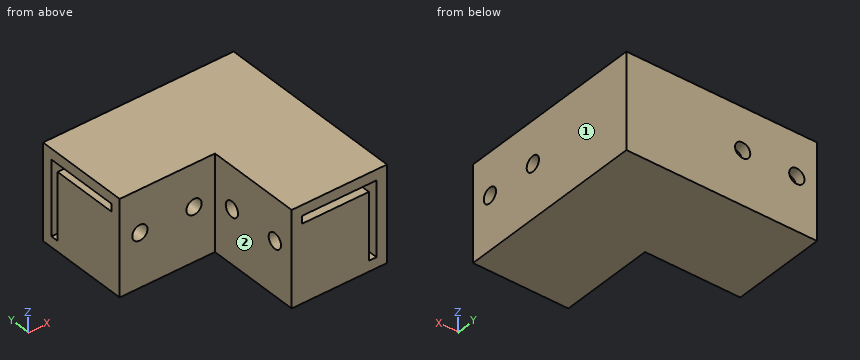
```python
from build123d import *

# Parameters (mm, degrees)
F0_W      = 25
F0_H      = 25
F1_DEPTH  = 25
F2_DEPTH  = 25
F3_DEPTH  = 25
F4_W      = 25
F4_H      = 25
F5_DEPTH  = 25
F6_W      = 17.5
F6_H      = 2
F6_W_2    = 2
F6_H_2    = 17.5
F7_DEPTH  = 25
F8_W      = 2
F8_H      = 2
F8_W_2    = 17.5
F8_H_2    = 17.5
F9_DEPTH  = 25
F10_R     = 2
F11_DEPTH = 25
F12_R     = 2
F13_DEPTH = 25


# Not quite as in the source:
# - a feature names something its author has since deleted; it is built from what else it names


with BuildPart() as f1:
    # F0 (on Top) → F1 (new body)
    with BuildSketch(Plane.XY):
        with Locations((12.5, 12.5)):
            Rectangle(F0_W, F0_H)
    extrude(amount=F1_DEPTH)

    # F2 (add): a face of the model
    f2_faces = [f1.faces().sort_by_distance(p)[0] for p in [
        (12.5, 0, 12.5),
    ]]
    extrude(f2_faces, amount=F2_DEPTH)

    # F3 (add): a face of the model
    f3_faces = [f1.faces().sort_by_distance(p)[0] for p in [
        (0, 0, 12.5),
    ]]
    extrude(f3_faces, amount=F3_DEPTH)

    # F4 (on face) → F5 (cut)
    with BuildSketch(Plane.XY.offset(25)):
        with Locations((-12.5, -12.5)):
            Rectangle(F4_W, F4_H)
    extrude(amount=-F5_DEPTH, mode=Mode.SUBTRACT)

    # F6 (on face) → F7 (cut)
    with BuildSketch(Plane.XZ.offset(25)):
        with Locations((11.5, 21.25)):
            Rectangle(F6_W, F6_H)
        with Locations((21.25, 21.25)):
            Rectangle(F6_W_2, F6_H)
        with Locations((21.25, 11.5)):
            Rectangle(F6_W_2, F6_H_2)
    extrude(amount=-F7_DEPTH, mode=Mode.SUBTRACT)

    # F8 (on face) → F9 (cut)
    with BuildSketch(Plane(origin=(-25, 0, 0), x_dir=(0, -1, 0), z_dir=(-1, 0, 0))):
        with Locations((-21.25, 21.25)):
            Rectangle(F8_W, F8_H)
        with Locations((-11.5, 21.25)):
            Rectangle(F8_W_2, F8_H)
        with Locations((-21.25, 11.5)):
            Rectangle(F8_W, F8_H_2)
    extrude(amount=-F9_DEPTH, mode=Mode.SUBTRACT)

    # F10 (on face) → F11 (cut)
    with BuildSketch(Plane(origin=(0, 25, 0), x_dir=(-1, 0, 0), z_dir=(0, 1, 0))):
        with Locations((19.7084973779, 14)):
            Circle(F10_R)
        with Locations((5.5, 14)):
            Circle(F10_R)
    extrude(amount=-F11_DEPTH, mode=Mode.SUBTRACT)

    # F12 (on face) → F13 (cut)
    with BuildSketch(Plane.YZ.offset(25)):
        with Locations((-19.5, 14)):
            Circle(F12_R)
        with Locations((-5.5, 14)):
            Circle(F12_R)
    extrude(amount=-F13_DEPTH, mode=Mode.SUBTRACT)


solid = f1.part
```
Work out the finished part from the listing and answer in its coordinate system (mm). Face numbers are marked on the shaded views. A direction names the side the tool comes from. Round coordinates to 2 decimals unless told otherwise and drop trailing zeros. Write each loop counter-clockwise with the first axis right and the second up, starting at its lowest first coordinate (ties: lowest second). Pieces come first, ordered by that corner, then holes. Notation, with made-up numbers: (84, 89.25) - (135, 89.25) arc R16 ccw to (135, 107.25) - close; hole circle Ø4 at (-21.75, 65.5). An arc over 180 degrees is marked (long way). Return JSON: item names as keys, results as strings. Group by question number.
Q1. The part is cut by section A-A on y = -19.5. Write down the section's boundary in (x, z), then the cut area to 3 significant figures.
Q2. The part is cut by section C-C on y = 17.5. Write down the section's boundary in (x, z).
Q3. Each of these flat-tipped pins is pushed along its axis until it touches: pin 1 Ø5 at (y, z) = (-11, 21) entering from -X; pin 2 Ø8 at (x, z) = (-17.5, 9.5) entering from -Y. Where does it stop, or does it pass through?
Q4. Find the intervals of material crossed by L1, parallel to Z at x = 8.5, y = -19.5; L2, parallel to Y at x = -22, z = 21.5; L3, parallel to X at y = -9, z = 15.5, in increasing order.
Q5. The part is cut by section D-D on x = 14. Write down the section's boundary in (y, z).
Q6. The part is cut by section B-B on x = -19. Write down the section's boundary in (y, z).
Q7. For the marked faces 1 and 2, determine the directions among +Z, -Z, +X, -X, +Y, -Y from which every point of the face is accessible in a straight line to the end or side of a thin tool.
Solved:
{
 "1": {"outline": "(0, 0) - (25, 0) - (25, 12) - (22.25, 12) - (22.25, 2.75) - (20.25, 2.75) - (20.25, 12) - (0, 12) - close; (0, 16) - (20.25, 16) - (20.25, 20.25) - (2.75, 20.25) - (2.75, 22.25) - (22.25, 22.25) - (22.25, 16) - (25, 16) - (25, 25) - (0, 25) - close", "area": "459 mm²"},
 "2": {"outline": "(-25, 0) - (25, 0) - (25, 25) - (-25, 25) - (-25, 22.25) - (0, 22.25) - (0, 20.25) - (-25, 20.25) - close; hole circle Ø4 at (-19.71, 14); hole circle Ø4 at (-5.5, 14)"},
 "3": {"pin 1": "x = 0", "pin 2": "y = 0"},
 "4": {"L1": "0 to 12, 16 to 20.25, 22.25 to 25", "L2": "0 to 2.75, 22.25 to 25", "L3": "0 to 20.25, 22.25 to 25"},
 "5": {"outline": "(-25, 0) - (25, 0) - (25, 25) - (-25, 25) - (-25, 22.25) - (0, 22.25) - (0, 20.25) - (-25, 20.25) - close; hole circle Ø4 at (-19.5, 14); hole circle Ø4 at (-5.5, 14)"},
 "6": {"outline": "(0, 0) - (25, 0) - (25, 12.13) - (22.25, 12.13) - (22.25, 2.75) - (20.25, 2.75) - (20.25, 12.13) - (0, 12.13) - close; (0, 15.87) - (20.25, 15.87) - (20.25, 20.25) - (2.75, 20.25) - (2.75, 22.25) - (22.25, 22.25) - (22.25, 15.87) - (25, 15.87) - (25, 25) - (0, 25) - close"},
 "7": {"face 1": "+Z, -Z, +X, +Y, -Y", "face 2": "+Z, -Z, -X, -Y"}
}
